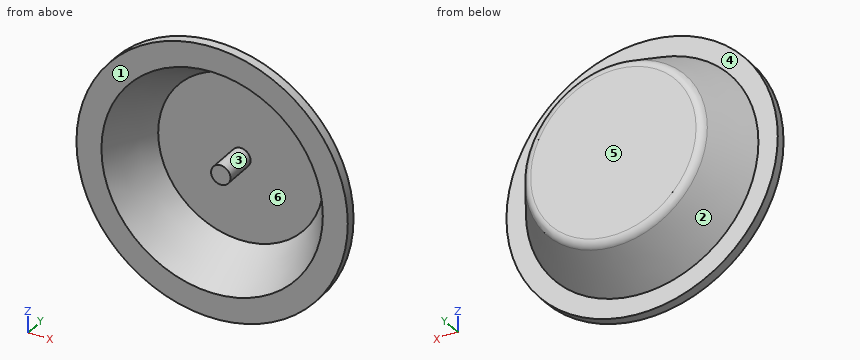
```python
from build123d import *


with BuildPart() as part:
    # Sketch1 → Revolve1 (revolve)
    with BuildSketch(Plane.XY):
        with BuildLine():
            Line((-35.56, 0), (-35.56, 2.54))
            Line((-35.56, 2.54), (-30.48, 2.54))
            Line((-30.48, 2.54), (-23.880886423, 13.97))
            ThreePointArc((-23.880886423, 13.97), (-22.951181898, 14.899704526), (-21.681181898, 15.24))
            Line((-21.681181898, 15.24), (0, 15.24))
            Line((0, 15.24), (0, 3.81))
            Line((0, 3.81), (-2.54, 3.81))
            Line((-2.54, 3.81), (-2.54, 12.7))
            Line((-2.54, 12.7), (-21.681181898, 12.7))
            Line((-21.681181898, 12.7), (-29.013530316, 0))
            Line((-29.013530316, 0), (-35.56, 0))
        make_face()
    revolve(axis=Axis((0, 15.24, 0), (0, -1, 0)))


solid = part.part
```
Here's how the part is built. I have some questions about the finished solid (model axes, mm). Face numbers are marked on the shaded views. A direction names the side the tool comes from. Round coordinates to 2 decimals unless told otherwise and drop trailing zeros. Write each loop counter-clockwise with the first axis right and the second up, starting at its lowest first coordinate (ties: lowest second). Pieces come first, ordered by that corner, then holes. Notation, with made-up numbers: M 85,-14 L 92,-14 A9 cw 92,-10 Z; hole C 81,20.25 d10. An arc over 180 degrees is marked long. Answer as CSV lines item,"result". Start each with the question number.
1. Suppose I cut it at A-A on x = 0. Write out the boundary of the cut face in (y, z).
2. Suppose I cut it at C-C on z = 0. Write out the boundary of the cut face in (x, y), then the cut area to 3 significant figures.
3. I need wall thicknesses on probe 1 along Y at (x, z) = (15, 28); probe 2 along Y at (x, z) = (1.5, 21); probe 3 along Z at (x, y) = (15, 6.25). Which ranges of each line are inside material? Lowest first, please.
4. Suppose I cut it at B-B on y = 6.5. Write out the boundary of the cut face in (x, z).
5. I'm going to push flat-ended pins straight in: pin 1 Ø5.5 at (x, z) = (0, -0.5) entering from -Y; pin 2 Ø2 at (y, z) = (11.5, -9) entering from +X; pin 3 Ø1.5 at (y, z) = (8.5, -0.5) entering from +X. Where does each tip first touch, or does it pass through?
6. Thinking about a two-plate mould opening in X: for the marked faces 1, 2 and 3, which applies, released by +X, released by -X, zero draft, split by the parting line, or undercut?
7. On a 3-axis mill with a long thin cutter (end or side, diameter ignored), from which of +Z, -Z, +X, -X, +Y, -Y can I reach the whole of each face in a straight line? I mean the marked faces 4, 5 and 6. Say none if no direction works.
Check result:
1,outline,"M 0,-35.56 L 2.54,-35.56 L 2.54,-30.48 L 13.97,-23.88 A2.54 ccw 15.24,-21.68 L 15.24,21.68 A2.54 ccw 13.97,23.88 L 2.54,30.48 L 2.54,35.56 L 0,35.56 L 0,29.01 L 12.7,21.68 L 12.7,2.54 L 3.81,2.54 L 3.81,-2.54 L 12.7,-2.54 L 12.7,-21.68 L 0,-29.01 Z"
2,outline,"M -35.56,0 L -29.01,0 L -21.68,12.7 L -2.54,12.7 L -2.54,3.81 L 2.54,3.81 L 2.54,12.7 L 21.68,12.7 L 29.01,0 L 35.56,0 L 35.56,2.54 L 30.48,2.54 L 23.88,13.97 A2.54 ccw 21.68,15.24 L -21.68,15.24 A2.54 ccw -23.88,13.97 L -30.48,2.54 L -35.56,2.54 Z"
2,area,"262 mm2"
3,probe 1,"y = 0 to 2.54"
3,probe 2,"y = 12.7 to 15.24"
3,probe 3,"z = -24.04 to -20.5, 20.5 to 24.04"
4,outline,"C 0,0 d56.39; C 0,0 d5.08; hole C 0,0 d50.52"
5,pin 1,"stops at y = 3.81"
5,pin 2,"stops at x = 24.37"
5,pin 3,"stops at x = 27.47"
6,face 1,"zero draft"
6,face 2,"split by the parting line"
6,face 3,"undercut"
7,face 4,"+Y"
7,face 5,"+Z, -Z, +X, -X, +Y"
7,face 6,"-Y"
